The listing builds one solid part. Answer for the finished solid, in the listing's coordinates (mm). A direction names the side the tool comes from. Round coordinates to 2 decimals unless told otherwise and drop trailing zeros. Loops run counter-clockwise (first coordinate to the right, second up) from the corner with the lowest first, then second, coordinate; pieces in that order, holes last. Notation, with made-up numbers: (-24, 63) -> (3, 63) arc R14 cw to (3, 70) -> close; hole circle Ø3 at (-5.5, 39). An arc over 180 degrees is marked (long way). Answer in a Markdown table with one row per item. Add a question column.
```python
from build123d import *

# Parameters (mm, degrees)
SKETCH1_W           = 4
SKETCH1_H           = 0.5
BOSS_EXTRUDE1_DEPTH = 5
SKETCH2_W           = 4
SKETCH2_H           = 2.5
BOSS_EXTRUDE2_DEPTH = 2
BOSS_EXTRUDE4_DEPTH = 4


with BuildPart() as part:
    # Sketch1 → Boss-Extrude1 (new body)
    with BuildSketch(Plane(origin=(0, 0, 0), x_dir=(1, 0, 0), z_dir=(0, 1, 0))):
        with Locations((2, 0.25)):
            Rectangle(SKETCH1_W, SKETCH1_H)
    extrude(amount=BOSS_EXTRUDE1_DEPTH)

    # Sketch2 → Boss-Extrude2 (add)
    with BuildSketch(Plane(origin=(0, 0, -0.5), x_dir=(-1, 0, 0), z_dir=(0, 0, -1))):
        with Locations((-2, 3.75)):
            Rectangle(SKETCH2_W, SKETCH2_H)
    extrude(amount=BOSS_EXTRUDE2_DEPTH)

    # Sketch4 → Boss-Extrude4 (add)
    with BuildSketch(Plane.ZY):
        Polygon((0, 5), (0, 0), (5, 0), align=None)
    extrude(amount=-BOSS_EXTRUDE4_DEPTH)


solid = part.part
```
Item 1: Consider L1, parallel to Y at x = 1.25, z = -1; L2, parallel to Y at x = 0.75, z = 2.5; L3, parallel to Z at x = 0.6, y = 3.1. Determine where each line is inside the solid, lowest interval first. Write a range as from..to.
Item 2: Section A-A, the plane y = 1.4 is taken. Write down the section's boundary in (x, z).
Item 3: Section C-C, the plane x = 0.3 is taken. Write down the section's boundary in (y, z), and give its area (3 significant figures).
Item 4: For faces 1 (the flat face through (0, 3, 0)), 2 (the flat face through (2, 2.5, -1)), determine the directions among +Z, -Z, +X, -X, +Y, -Y from which every point of the face is accessible in a straight line to the end or side of a thin tool.
Item 5: Section B-B, the plane z = 0.5 is taken. Write down the section's boundary in (x, y).
Item 6: Flat-ended cylindrical pins translate along their axes: P1, Ø2, axis at x = 3, y = 1, coming from the -Z side; P2, Ø1, axis at x = 1, y = 4, coming from the +Z side; P3, Ø2, axis at x = 3, z = -2, coming from the -Y side. Find the tip coordinate at first contact, or state that the pin passes through.
Here are the results:
| question | item | result |
|---|---|---|
| 1 | L1 | y = 2.5..5 |
| 1 | L2 | y = 0..2.5 |
| 1 | L3 | z = -2.5..1.9 |
| 2 | outline | (0, -0.5) -> (4, -0.5) -> (4, 3.6) -> (0, 3.6) -> close |
| 3 | outline | (0, -0.5) -> (2.5, -0.5) -> (2.5, -2.5) -> (5, -2.5) -> (5, 0) -> (0, 5) -> close |
| 3 | area | 20.0 mm² |
| 4 | face 1 | +Z, -Z, -X, +Y, -Y |
| 4 | face 2 | -Z, +X, -X, -Y |
| 5 | outline | (0, 0) -> (4, 0) -> (4, 4.5) -> (0, 4.5) -> close |
| 6 | P1 | stops at z = -0.5 |
| 6 | P2 | stops at z = 1.5 |
| 6 | P3 | stops at y = 2.5 |
